Build history of the part. All positions in model axes, mm. Face numbers are marked on the shaded views. A direction names the side the tool comes from. Coordinates: 2 decimals unless noted, no trailing zeros. Order: outer loops, then holes, each group sorted by start corner. A loop starts at its lowest first (then second) coordinate and runs counter-clockwise, first axis right, second up. Notation, with made-up numbers: (74.25, 37) -> (117.25, 37) arc R27 ccw to (117.25, 60) -> close; hole circle Ø8 at (40.5, 78.5). An arc over 180 degrees is marked (long way). Write each question's results on one line, items separated by ' | '.
from build123d import *
from build123d.topology import SkipClean

# Parameters (mm, degrees)
CUT_SWEEP1_PITCH = 1.5875
CUT_SWEEP1_TO    = 16.6878


with BuildPart() as part:
    # Sketch1 → Revolve1 (revolve)
    with BuildSketch(Plane.XY, mode=Mode.PRIVATE) as revolve1_sk:
        Polygon((-15.4686, 12.3444), (-15.4686, 11.176), (-7.227253544, 4.9657), (15.4686, 4.9657), (15.4686, 5.710555), (15.4686, 9.525), (10.406660515, 9.525), (-1.2192, 9.525), (-1.2192, 10.4902), (-8.7122, 10.4902), (-8.7122, 12.3444), align=None)
    revolve(revolve1_sk.sketch.rotate(Axis((-15.4686, 0, 0), (1, 0, 0)), 90), axis=Axis((-15.4686, 0, 0), (1, 0, 0)))

    # Cut-Sweep1: arcs per turn and ends read off the stored shape
    # Cut-Sweep1: the profile of Sketch4 profile screwed along a right-hand helix through 12.5 turns, 8 arcs to a turn; built about Z, then put on its axis
    cut_sweep1_z = Axis((0, 0, 0), (0, 0, 1))
    cut_sweep1_corners = [(9.5253, 0, -1.587326795), (9.5253, 0, -2.976735705), (8.493888504, 0, -2.38125), (8.493888504, 0, -2.1828125)]
    with BuildLine(mode=Mode.PRIVATE) as cut_sweep1_profile:
        Line(cut_sweep1_corners[0], cut_sweep1_corners[1])
        Line(cut_sweep1_corners[1], cut_sweep1_corners[2])
        Line(cut_sweep1_corners[2], cut_sweep1_corners[3])
        Line(cut_sweep1_corners[3], cut_sweep1_corners[0])
    cut_sweep1_cap = Face(cut_sweep1_profile.wire())
    cut_sweep1_turn_angles = [0, 22.5, 45, 67.5, 90, 112.5, 135, 157.5, 180, 202.5, 225, 247.5, 270, 292.5, 315, 337.5, 360]
    cut_sweep1_turn_weights = [1, 0.9238795325112867, 1, 0.9238795325112867, 1, 0.9238795325112867, 1, 0.9238795325112867, 1, 0.9238795325112867, 1, 0.9238795325112867, 1, 0.9238795325112867, 1, 0.9238795325112867, 1]
    cut_sweep1_turn_rails = [Edge.make_bspline([Vector(p[0], p[1], 0).rotate(cut_sweep1_z, cut_sweep1_turn_angles[k]) / cut_sweep1_turn_weights[k] + Vector(0, 0, p[2] + CUT_SWEEP1_PITCH * cut_sweep1_turn_angles[k] / 360) for k in range(17)], [0, 0, 0, 1, 1, 2, 2, 3, 3, 4, 4, 5, 5, 6, 6, 7, 7, 8, 8, 8], 2, cut_sweep1_turn_weights) for p in cut_sweep1_corners]
    cut_sweep1_turn_sides = [Face.make_surface_from_curves(cut_sweep1_turn_rails[p[0]], cut_sweep1_turn_rails[p[1]]) for p in [(0, 1), (1, 2), (2, 3), (3, 0)]]
    cut_sweep1_last_angles = [4320, 4342.5, 4365, 4387.5, 4410, 4432.5, 4455, 4477.5, 4500]
    cut_sweep1_last_weights = [1, 0.9238795325112867, 1, 0.9238795325112867, 1, 0.9238795325112867, 1, 0.9238795325112867, 1]
    cut_sweep1_last_rails = [Edge.make_bspline([Vector(p[0], p[1], 0).rotate(cut_sweep1_z, cut_sweep1_last_angles[k]) / cut_sweep1_last_weights[k] + Vector(0, 0, p[2] + CUT_SWEEP1_PITCH * cut_sweep1_last_angles[k] / 360) for k in range(9)], [0, 0, 0, 1, 1, 2, 2, 3, 3, 4, 4, 4], 2, cut_sweep1_last_weights) for p in cut_sweep1_corners]
    cut_sweep1_last_sides = [Face.make_surface_from_curves(cut_sweep1_last_rails[p[0]], cut_sweep1_last_rails[p[1]]) for p in [(0, 1), (1, 2), (2, 3), (3, 0)]]
    cut_sweep1 = Plane(origin=(15.4686, 0, 0), x_dir=(0, 1, 0), z_dir=(-1, 0, 0)) * split(Solid(Shell([*[p.moved(Location((0, 0, CUT_SWEEP1_PITCH * i))) for i in range(12) for p in cut_sweep1_turn_sides], *cut_sweep1_last_sides, cut_sweep1_cap, cut_sweep1_cap.rotate(cut_sweep1_z, 4500).moved(Location((0, 0, CUT_SWEEP1_PITCH * 4500 / 360)))])), bisect_by=Plane.XY.offset(CUT_SWEEP1_TO), keep=Keep.BOTTOM, mode=Mode.PRIVATE)
    add(cut_sweep1, mode=Mode.SUBTRACT)

    # Sketch5 → Cut-Revolve1 (revolve, cut)
    with BuildSketch(Plane.XY, mode=Mode.PRIVATE) as cut_revolve1_sk:
        Polygon((15.4686, 5.710555), (11.842405564, 8.443088504), (10.254905564, 8.443088504), (9.172994068, 9.525), (15.4686, 9.525), align=None)
        Polygon((-1.2192, 9.525), (-1.2192, 8.443088504), (0.3683, 8.443088504), (1.450211496, 9.525), align=None)
    revolve(cut_revolve1_sk.sketch.rotate(Axis((0, 0, 0), (-1, 0, 0)), 90), axis=Axis((0, 0, 0), (-1, 0, 0)), mode=Mode.SUBTRACT)

    # Revolve2: read off the stored shape, not the designer's step
    # Revolve2 outline → Revolve2 (revolve)
    with SkipClean():  # the faces are left unmerged after this step: merging them gives an invalid solid
        with BuildSketch(Plane.YX):
            Polygon((9.525, 1.450211496), (9.525, 9.172994068), (8.443088504, 10.254905564), (8.443088504, 0.3683), align=None)
        revolve(axis=Axis((0, 0, 0), (1, 0, 0)))


solid = part.part
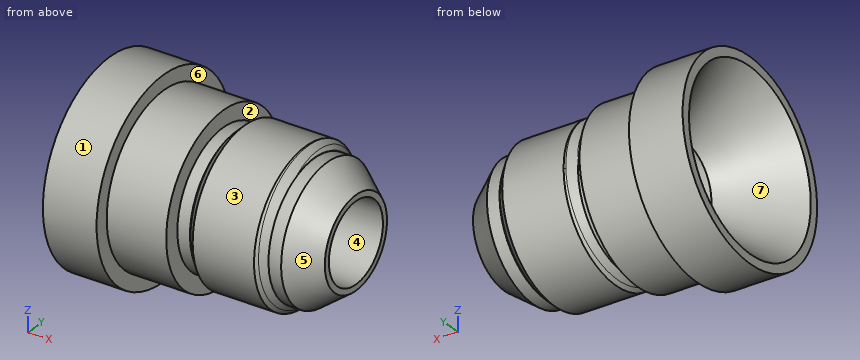
Item 1: Pull direction Y, two halves, no side cores. Call the marked faces 4, 5, 6 and 7: released by +Y, released by -Y, zero draft, split by the parting line, or undercut.
Answer:
face 4: undercut | face 5: split by the parting line | face 6: zero draft | face 7: undercut
Item 2: Tool access for the marked faces 1, 2 and 3: list every direction of +Z, -Z, +X, -X, +Y, -Y with a clear straight run to the whole face (end or side of a thin tool).
Answer:
face 1: +X, -X | face 2: none | face 3: +X
Item 3: Drill centre lines: line 1 (Y direction, x = 11, z = 0); line 2 (Y direction, x = 7, z = 0) (3 decimals); line 3 (Z direction, x = -10, y = -0.75). Where is each one in solid material? Low to high. Write a range as from..to.
Answer:
line 1: y = -8.44..-4.97, 4.97..8.44 | line 2: y = -9.525..-4.966, 4.966..9.525 | line 3: z = -12.32..-7.02, 7.02..12.32
Item 4: Slice it at B-B, the plane x = 6. List the corners of the cut face in (y, z) (3 decimals).
Answer:
outline: circle Ø19.05 at (0, 0); hole circle Ø9.931 at (0, 0)
Item 5: Slice it at A-A, the plane x = -2.5. List the corners of the cut face in (y, z), and give its area (3 significant figures).
Answer:
outline: circle Ø20.98 at (0, 0); hole circle Ø9.93 at (0, 0) | area: 268 mm^2
Item 6: Pin check, flat tips, straight feed: pin 1 (3 mm diameter, centred on x = -3.5, y = -3.5, fed in from -Z); pin 2 (4 mm diameter, centred on x = 6.5, y = 4, fed in from -Z); pin 3 (2 mm diameter, centred on x = -12, z = -7.5, fed in from +Y); pin 4 (8 mm diameter, centred on y = -0.5, z = 8.5, fed in from -X). Stop position of each tip, or through.
Answer:
pin 1: stops at z = -10.3 | pin 2: stops at z = -9.31 | pin 3: stops at y = 10.49 | pin 4: stops at x = -15.47
